The listing builds one solid part. Answer for the finished solid, in the listing's coordinates (mm). Face numbers are marked on the shaded views. A direction names the side the tool comes from. Give positions to 0.01 mm unless a question says otherwise; leave off trailing zeros. Order: outer loops, then holes, each group sorted by start corner. A loop starts at its lowest first (then second) coordinate and runs counter-clockwise, first axis right, second up. Notation, with made-up numbers: (22.5, -2.5) - (80.5, -2.5) arc R17 cw to (80.5, 24.5) - close; hole circle Ø8 at (-1, 75). An arc over 180 degrees is marked (long way). Write each question's results on one line, items separated by ' | '. Start each with the question number.
1. Section D-D (z = 148.5) is taken. Give the vertices of the cut face in (x, y), and give its area (3 significant figures).
2. Section A-A (z = 48) is taken. Give the vertices of the cut face in (x, y), and give its area (3 significant figures).
3. Which of the six approach directions +Z, -Z, +X, -X, +Y, -Y give full straight-line access (tool end or side, diameter ignored) to the marked faces 4, 5 and 6?
4. Section B-B (x = -37) is taken. Give the vertices of the cut face in (y, z), and give its area (3 significant figures).
5. Find the intervals of material crossed by L1, parallel to X at y = 182, z = 86.5; L2, parallel to Y at x = -71.5, z = 102; L3, parallel to Y at x = 25.5, z = 237, in increasing order.
6. Determine the mould class of the marked faces 1, 2 and 3 for opening direction Y: released by +Y, released by -Y, zero draft, split by the parting line, or undercut.
7. Section C-C (y = -2) is taken. Give the vertices of the cut face in (x, z), and give its area (4 significant figures).
8. Flat-ended cylindrical pins translate along their axes: pin 1 (2 mm diameter, centred on y = -257.5, z = 78, fed in from +X); pin 2 (1.5 mm diameter, centred on x = -120.5, y = 143, fed in from -Z); pin 3 (3 mm diameter, centred on x = -194, y = -175, fed in from +Z); pin 4 (1 mm diameter, centred on x = -123.5, z = 51.5, fed in from -Y). Find the tip coordinate at first contact, or state that the pin passes through.
from build123d import *

# Parameters (mm, degrees)
F0_W     = 304.8
F0_H     = 406.4
F1_DEPTH = 254
F2_T     = -12.7
F3_R     = 76.2
F4_DEPTH = 152.4


with BuildPart() as f1:
    # F0 (on Top) → F1 (new body)
    with BuildSketch(Plane.XY):
        with Locations((-92.487486, 36.538938)):
            Rectangle(F0_W, F0_H)
    extrude(amount=F1_DEPTH)

    # F2
    f2_openings = [f1.faces().sort_by_distance(p)[0] for p in [
        (-92.487486, 36.538938, 254),
    ]]
    offset(amount=F2_T, openings=f2_openings)

    # F3 (on face) → F4 (join)
    with BuildSketch(Plane.XZ.offset(166.661062)):
        with Locations((-131.477997, 138.828054)):
            Circle(F3_R)
    extrude(amount=F4_DEPTH)


solid = f1.part
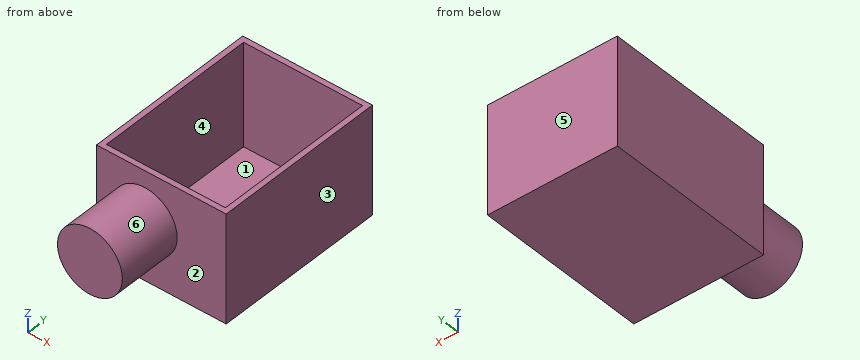
Reported:
1) outline: (-244.89, -166.66) - (-207.06, -166.66) - (-207.06, -319.06) - (-55.89, -319.06) - (-55.89, -166.66) - (59.91, -166.66) - (59.91, 239.74) - (-244.89, 239.74) - close; hole (-232.19, -153.96) - (47.21, -153.96) - (47.21, 227.04) - (-232.19, 227.04) - close | area: 40,500 mm²
2) outline: (-244.89, -166.66) - (59.91, -166.66) - (59.91, 239.74) - (-244.89, 239.74) - close; hole (-232.19, -153.96) - (47.21, -153.96) - (47.21, 227.04) - (-232.19, 227.04) - close | area: 17,400 mm²
3) face 4: +Z | face 5: +Z, -Z, +X, -X, +Y | face 6: -Y
4) outline: (-166.66, 0) - (239.74, 0) - (239.74, 254) - (227.04, 254) - (227.04, 12.7) - (-153.96, 12.7) - (-153.96, 254) - (-166.66, 254) - close | area: 11,300 mm²
5) L1: -244.89 to -232.19, 47.21 to 59.91 | L2: -319.06 to -153.96, 227.04 to 239.74 | L3: -166.66 to -153.96, 227.04 to 239.74
6) face 1: undercut | face 2: released by -Y | face 3: zero draft
7) outline: (-244.89, 0) - (59.91, 0) - (59.91, 254) - (47.21, 254) - (47.21, 12.7) - (-232.19, 12.7) - (-232.19, 254) - (-244.89, 254) - close | area: 10,000 mm²
8) pin 1: x = -84.29 | pin 2: z = 0 | pin 3: z = 184.47 | pin 4: y = -166.66
